Source: CAD feature listing. Evaluate the final solid. Frame: model axes, mm. Face numbers are marked on the shaded views. A direction names the side the tool comes from. Give positions to 0.01 mm unless a question says otherwise; leave off trailing zeros. Order: outer loops, then holes, each group sorted by start corner. A loop starts at its lowest first (then second) coordinate and runs counter-clockwise, first axis right, second up.
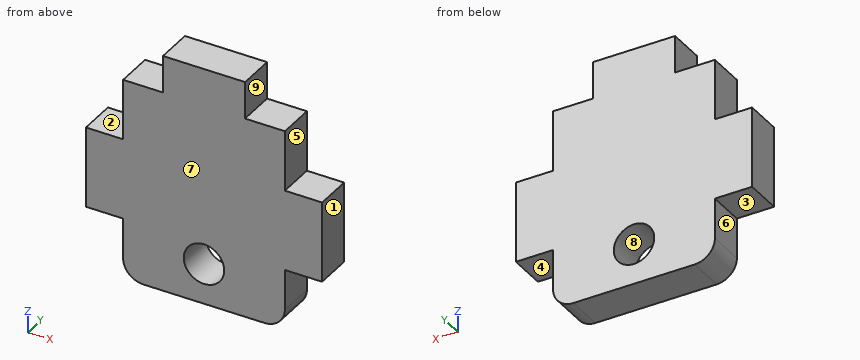
```python
from build123d import *

# Parameters (mm, degrees)
F0_R     = 3.175
F1_DEPTH = 5.842
F2_R     = 3.175


with BuildPart() as f1:
    # F0 (on Front) → F1 (new body)
    with BuildSketch(Plane.XZ):
        Polygon((-12.7, 3.175), (-12.7, -6.35), (12.7, -6.35), (12.7, 3.175), (18.542, 3.175), (18.542, 15.875), (12.7, 15.875), (12.7, 25.4), (6.45, 25.4), (6.45, 31.242), (-6.45, 31.242), (-6.45, 25.4), (-12.7, 25.4), (-12.7, 15.875), (-18.542, 15.875), (-18.542, 3.175), align=None)
        Circle(F0_R, mode=Mode.SUBTRACT)
    extrude(amount=F1_DEPTH)

    # F2
    f2_edges = [f1.edges().sort_by_distance(p)[0] for p in [
        (-12.7, -2.921, -6.35),
        (12.7, -2.921, -6.35),
    ]]
    fillet(f2_edges, radius=F2_R)


solid = f1.part
```
1) Section query B-B, the plane x = 0. Return the cut outline in (y, z) (3 decimals), and give its area (3 significant figures).
Report:
outline: (-5.842, -6.35) - (0, -6.35) - (0, -3.175) - (-5.842, -3.175) - close; (-5.842, 3.175) - (0, 3.175) - (0, 31.242) - (-5.842, 31.242) - close
area: 183 mm2
2) Pin query (flat end, axial travel): pin 1 (1.8 mm diameter, centred on y = -1.5, z = 0, fed in from +X); pin 2 (3 mm diameter, centred on x = 14.5, y = -3, fed in from -Z) (3 decimals); pin 3 (5 mm diameter, centred on x = -5, z = 8.5, fed in from +Y); pin 4 (3 mm diameter, centred on y = -4.5, z = -1, fed in from -X). Return the tip coordinate at first contact, or that it passes through.
Report:
pin 1: stops at x = 12.7
pin 2: stops at z = 3.175
pin 3: stops at y = 0
pin 4: stops at x = -12.7
3) Reachability of the marked faces 1, 2, 3, 4 and 5 from +Z, -Z, +X, -X, +Y, -Y: full face, straight path, thin tool, end or side. Return the list, or none.
Report:
face 1: +Z, -Z, +X, +Y, -Y
face 2: +Z, -X, +Y, -Y
face 3: -Z, -X, +Y, -Y
face 4: -Z, +X, +Y, -Y
face 5: +Z, +X, +Y, -Y
4) Material intervals for L1, parallel to Z at x = 0, y = -3.4 (3 decimals); L2, parallel to Z at x = -9.5, y = -5.55; L3, parallel to X at y = -1.9, z = 18.5, sorted ascending.
Report:
L1: z = -6.35 to -3.175, 3.175 to 31.242
L2: z = -6.35 to 25.4
L3: x = -12.7 to 12.7
5) Section query C-C, the plane y = -1.9. Return the cut outline in (x, z) (3 decimals).
Report:
outline: (-18.542, 3.175) - (-12.7, 3.175) - (-12.7, -3.175) arc R3.175 ccw to (-9.525, -6.35) - (9.525, -6.35) arc R3.175 ccw to (12.7, -3.175) - (12.7, 3.175) - (18.542, 3.175) - (18.542, 15.875) - (12.7, 15.875) - (12.7, 25.4) - (6.45, 25.4) - (6.45, 31.242) - (-6.45, 31.242) - (-6.45, 25.4) - (-12.7, 25.4) - (-12.7, 15.875) - (-18.542, 15.875) - close; hole circle Ø6.35 at (0, 0)
6) Draft query along X for the marked faces 6, 7, 8 and 9. Return one class per face: +X half, -X half, draft (parallel to the pull), parting line (faces both ways), or undercut.
Report:
face 6: -X half
face 7: draft
face 8: undercut
face 9: +X half
7) Section query A-A, the plane z = 0. Return the cut outline in (x, y) (3 decimals), and give its area (3 significant figures).
Report:
outline: (-12.7, -5.842) - (-3.175, -5.842) - (-3.175, 0) - (-12.7, 0) - close; (3.175, -5.842) - (12.7, -5.842) - (12.7, 0) - (3.175, 0) - close
area: 111 mm2
8) Section query D-D, the plane z = 21. Return the cut outline in (x, y).
Report:
outline: (-12.7, -5.84) - (12.7, -5.84) - (12.7, 0) - (-12.7, 0) - close
